Verification items for the finished model (mm, model axes). A direction names the side the tool comes from. Round coordinates to 2 decimals unless told otherwise and drop trailing zeros. Write each loop counter-clockwise with the first axis right and the second up, starting at its lowest first coordinate (ties: lowest second). Pieces come first, ordered by that corner, then holes. Notation, with made-up numbers: (0, 67) -> (6, 67) arc R27 cw to (6, 87) -> close; hole circle Ø8 at (81.5, 55). An arc over 180 degrees is marked (long way). Answer as a JSON object with one key per item and string values. Group by question number.
(1) Sectioned sample at D-D on x = 23. Record the cut outline in (y, z), and give its area (3 significant figures).
(2) Draft check along Z on faces 1 (the face through (39, -25.4, -2)), 2 (the face through (-28.57, -25.04, 0.63)), 3 (the face through (-16, -38, -4.762)). Enter one of: released by +Z, released by -Z, zero draft, split by the parting line, or undercut.
(3) Gauge pin test, flat ends, axial feed: pin 1 Ø6 at (x, y) = (-17, -36) entering from -Z; pin 2 Ø2 at (x, y) = (-18, -34) entering from +Z; pin 3 Ø10 at (x, y) = (35, -20) entering from -Z; pin 4 Ø8 at (x, z) = (61, 6) entering from -Y. Record the tip position at first contact, or that the pin passes through.
(4) Sectioned sample at B-B on y = -23. Count the separate pieces of the cut face and the enclosed holes in it, and give its area (3 significant figures).
(5) Sectioned sample at A-A on x = 44.5. Record the cut outline in (y, z), and give its area (3 significant figures).
(6) Set-up check for faces 4 (the face through (-19.05, -38, 0)), 5 (the face through (19.05, -25, 0)), 6 (the face through (22, 0, 0)): record each of +Z, -Z, +X, -X, +Y, -Y from which the full face is reachable in a straight line by a thin tool's end or side.
(7) Scan lines: L1, parallel to X at y = -6, z = -5; L2, parallel to Z at x = 54, y = -23; L3, parallel to Z at x = 12.5, y = -19. Record each from-to range of solid material in increasing order. Write a range as from..to.
```python
from build123d import *

# Parameters (mm, degrees)
F0_R     = 14.2875
F1_DEPTH = 25.4
F2_DEPTH = 50.8


with BuildPart() as f1:
    # F0 (on Front) → F1 (new body)
    with BuildSketch(Plane.XZ):
        with BuildLine():
            Line((9.8852824268, 26.8106660929), (0, 28.575))
            ThreePointArc((0, 28.575), (-28.575, 0), (0, -28.575))
            Line((0, -28.575), (9.7880218685, -26.8463266184))
            ThreePointArc((9.7880218685, -26.8463266184), (23.4117849586, -16.3834962707), (28.575, 0))
            ThreePointArc((28.575, 0), (23.4414437519, 16.3410323978), (9.8852824268, 26.8106660929))
        make_face()
        with BuildLine():
            ThreePointArc((-13.4703841816, 4.7625), (0, 14.2875), (13.4703841816, 4.7625))
            Line((13.4703841816, 4.7625), (19.05, 4.7625))
            Line((19.05, 4.7625), (19.05, -4.7625))
            Line((19.05, -4.7625), (13.4703841816, -4.7625))
            ThreePointArc((13.4703841816, -4.7625), (0, -14.2875), (-13.4703841816, -4.7625))
            Line((-13.4703841816, -4.7625), (-19.05, -4.7625))
            Line((-19.05, -4.7625), (-19.05, 4.7625))
            Line((-19.05, 4.7625), (-13.4703841816, 4.7625))
        make_face(mode=Mode.SUBTRACT)
        with BuildLine():
            Line((53.4134443953, 19.0417214375), (9.8852824268, 26.8106660929))
            ThreePointArc((9.8852824268, 26.8106660929), (23.4414437519, 16.3410323978), (28.575, 0))
            ThreePointArc((28.575, 0), (23.4117849586, -16.3834962707), (9.7880218685, -26.8463266184))
            Line((9.7880218685, -26.8463266184), (53.9323258703, -19.0499522025))
            ThreePointArc((53.9323258703, -19.0499522025), (34.9267671799, -0.2594733756), (53.4134443953, 19.0417214375))
        make_face()
        with BuildLine():
            ThreePointArc((73.025, 0), (67.2453591837, 13.6674821066), (53.4134443953, 19.0417214375))
            ThreePointArc((53.4134443953, 19.0417214375), (34.9267671799, -0.2594733756), (53.9323258703, -19.0499522025))
            ThreePointArc((53.9323258703, -19.0499522025), (67.4302881394, -13.4854633248), (73.025, 0))
        make_face()
        with Locations((53.975, 0)):
            Circle(F0_R, mode=Mode.SUBTRACT)
        with BuildLine():
            ThreePointArc((-13.4703841816, -4.7625), (-14.2875, 0), (-13.4703841816, 4.7625))
            Line((-13.4703841816, 4.7625), (-19.05, 4.7625))
            Line((-19.05, 4.7625), (-19.05, -4.7625))
            Line((-19.05, -4.7625), (-13.4703841816, -4.7625))
        make_face()
    extrude(amount=F1_DEPTH)

    # F0 (on Front) → F2 (join)
    with BuildSketch(Plane.XZ):
        with BuildLine():
            Line((9.8852824268, 26.8106660929), (0, 28.575))
            ThreePointArc((0, 28.575), (-28.575, 0), (0, -28.575))
            Line((0, -28.575), (9.7880218685, -26.8463266184))
            ThreePointArc((9.7880218685, -26.8463266184), (23.4117849586, -16.3834962707), (28.575, 0))
            ThreePointArc((28.575, 0), (23.4414437519, 16.3410323978), (9.8852824268, 26.8106660929))
        make_face()
        with BuildLine():
            ThreePointArc((-13.4703841816, 4.7625), (0, 14.2875), (13.4703841816, 4.7625))
            Line((13.4703841816, 4.7625), (19.05, 4.7625))
            Line((19.05, 4.7625), (19.05, -4.7625))
            Line((19.05, -4.7625), (13.4703841816, -4.7625))
            ThreePointArc((13.4703841816, -4.7625), (0, -14.2875), (-13.4703841816, -4.7625))
            Line((-13.4703841816, -4.7625), (-19.05, -4.7625))
            Line((-19.05, -4.7625), (-19.05, 4.7625))
            Line((-19.05, 4.7625), (-13.4703841816, 4.7625))
        make_face(mode=Mode.SUBTRACT)
    extrude(amount=F2_DEPTH)


solid = f1.part
```
Computed values:
{
 "1": {"outline": "(-50.8, -16.96) -> (-25.4, -16.96) -> (-25.4, -24.51) -> (0, -24.51) -> (0, 24.47) -> (-25.4, 24.47) -> (-25.4, 16.96) -> (-50.8, 16.96) -> close", "area": "2,110 mm2"},
 "2": {"face 1": "zero draft", "face 2": "split by the parting line", "face 3": "undercut"},
 "3": {"pin 1": "z = -24.91", "pin 2": "z = 22.97", "pin 3": "z = -23.28", "pin 4": "through"},
 "4": {"separate pieces": "1", "enclosed holes": "2", "area": "3,090 mm2"},
 "5": {"outline": "(-25.4, -20.72) -> (0, -20.72) -> (0, -10.69) -> (-25.4, -10.69) -> close; (-25.4, 10.69) -> (0, 10.69) -> (0, 20.63) -> (-25.4, 20.63) -> close", "area": "507 mm2"},
 "6": {"face 4": "-Y", "face 5": "+Y, -Y", "face 6": "+Z, -Z, +X, -X, +Y"},
 "7": {"L1": "-28.13..-13.38, 13.38..40.59, 67.36..72.36", "L2": "-19.05..-14.29, 14.29..19.05", "L3": "-26.37..-6.92, 6.92..26.34"}
}
